Study the drawing (mm; zero at the part's minimum x, y, z) and answer. Give positions to 0.01 mm unless a question says otherwise; leave off trailing zeros. Loops run counter-clockwise (first coordinate to the right, second up) from the corner with the lowest first, then second, coordinate; pieces in that order, holes last. Notation, with made-up numbers: (49, 18) - (61, 18) arc R6 ccw to (61, 28) - close; hole circle Ø7 at (-21.75, 15). An arc over 180 degrees is marked (long way). Write item = value, one per line. Start each with the question number.
1) The part is cut by section C-C on y = 387. Write down the section's boundary in (x, z) (3 decimals).
2) The part is cut by section A-A on z = 48.5. Write down the section's boundary in (x, y), plus the area to 3 significant figures.
3) The part is cut by section B-B on x = 8.5. Write down the section's boundary in (y, z).
4) Consider probe 1 along Y at (x, z) = (31.75, 60.9) (3 decimals); probe 2 along Z at (x, y) = (31.5, 304.5); probe 3 along Y at (x, z) = (1, 31). Determine where each line is inside the solid, lowest interval first.
5) Flat-ended cylindrical pins translate along their axes: P1, Ø8.5, axis at x = 31.75, y = 355.6, coming from the +Z side; P2, Ø12, axis at x = 20, y = 112.5, coming from the -Z side (3 decimals); P3, Ø5, axis at x = 10, y = 310, coming from the -Z side; P4, Ø5.5, axis at x = 31.75, y = 488.95, coming from the -Z side. Find the tip coordinate at first contact, or state that the pin passes through.
6) The mould has two halves that part along X. Classify the marked faces 1 and 2: +X half, -X half, draft (parallel to the pull), parting line (faces both ways), or undercut.
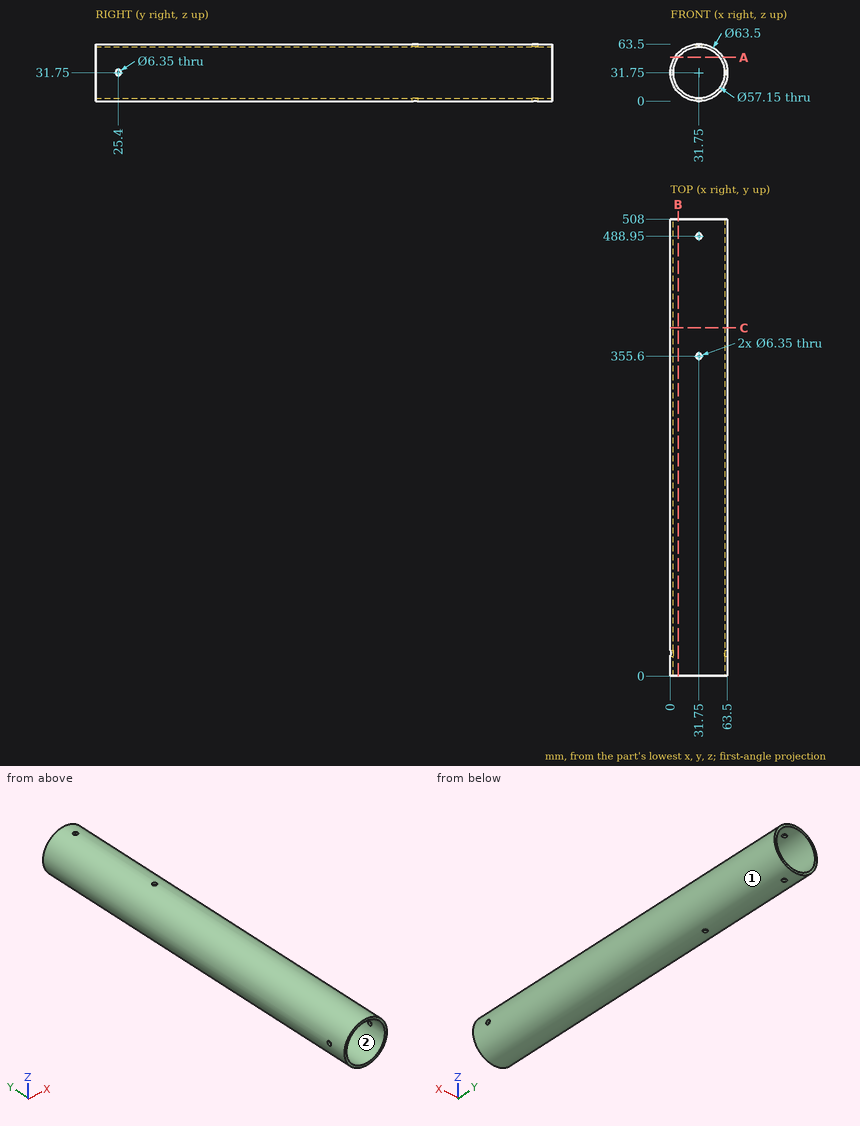
Answer below:
q1.outline = circle Ø63.5 at (31.75, 31.75); hole circle Ø57.15 at (31.75, 31.75)
q2.outline = (4.78, 0) - (8.6, 0) - (8.6, 508) - (4.78, 508) - close; (54.9, 0) - (58.72, 0) - (58.72, 508) - (54.9, 508) - close
q2.area = 3,880 mm2
q3.outline = (0, 10.13) - (508, 10.13) - (508, 15.14) - (0, 15.14) - close; (0, 48.36) - (508, 48.36) - (508, 53.37) - (0, 53.37) - close
q4.probe_1 = 0 to 352.425, 358.775 to 485.775, 492.125 to 508
q4.probe_2 = 0 to 3.18, 60.32 to 63.5
q4.probe_3 = 0 to 22.31, 28.49 to 508
q5.P1 = 63.5
q5.P2 = 0.525
q5.P3 = 6.5
q5.P4 = through
q6.face_1 = parting line
q6.face_2 = undercut
